```python
from build123d import *

# Parameters (mm, degrees)
SKETCH1_R           = 4.826
SKETCH1_R_2         = 4.064
SKETCH3_R           = 4.826
BOSS_EXTRUDE1_DEPTH = 2.54
BOSS_EXTRUDE1_DRAFT = -37
SKETCH5_R           = 4.826
BOSS_EXTRUDE2_DEPTH = 2.54
BOSS_EXTRUDE2_DRAFT = -37


with BuildPart() as part:
    # Sweep1: sweep along a path in Sketch2
    with BuildLine(Plane.XY) as sweep1_path:
        Line((0, 0), (0, 12.7))
        ThreePointArc((0, 12.7), (1.450094906, 19.990119387), (5.579615818, 26.170384182))
        Line((5.579615818, 26.170384182), (10.295384182, 30.886152545))
        ThreePointArc((10.295384182, 30.886152545), (15.875, 44.356536726), (10.295384182, 57.826920908))
        Line((10.295384182, 57.826920908), (5.579615818, 62.542689271))
        ThreePointArc((5.579615818, 62.542689271), (1.450094906, 68.722954066), (0, 76.013073453))
        Line((0, 76.013073453), (0, 88.713073453))
    # Sketch1 → Sweep1 (sweep)
    with BuildSketch(Plane(origin=(0, 0, 0), x_dir=(1, 0, 0), z_dir=(0, 1, 0))):
        Circle(SKETCH1_R)
        Circle(SKETCH1_R_2, mode=Mode.SUBTRACT)
    sweep(path=sweep1_path.line)


with BuildPart() as boss_extrude1_tool:
    # Sketch3 → Boss-Extrude1 (with draft: the straight prism first)
    with BuildSketch(Plane.XZ):
        with Locations(Location((0, 0, 0), (0, 0, 180))):
            Circle(SKETCH3_R)
    extrude(amount=BOSS_EXTRUDE1_DEPTH)
    # Boss-Extrude1: the draft: its side faces are tilted about the plane it starts from
    boss_extrude1_sides = [boss_extrude1_tool.faces().sort_by_distance(p)[0] for p in [
        (4.826, -1.27, 0),
    ]]
    draft(boss_extrude1_sides, Plane.XZ, BOSS_EXTRUDE1_DRAFT)


with BuildPart() as part_1:
    add(part.part)

    # Boss-Extrude1: add boss_extrude1_tool
    add(boss_extrude1_tool.part)

    # Cut-Extrude1 cone 1 section (through the dimple's axis) → Cut-Extrude1 (revolve, cut)
    with BuildSketch(Plane(origin=(0, -2.54, 0), x_dir=(0, 0, -1), z_dir=(1, 0, 0))):
        Polygon((0, 0), (5.978027287, 0), (0, 7.933110155), align=None)
    revolve(axis=Axis((0, -2.54, 0), (0, 1, 0)), mode=Mode.SUBTRACT)


with BuildPart() as boss_extrude2_tool:
    # Sketch5 → Boss-Extrude2 (with draft: the straight prism first)
    with BuildSketch(Plane(origin=(0, 88.713073453, 0), x_dir=(0, 0, -1), z_dir=(0, 1, 0))):
        with Locations(Location((0, 0, 0), (0, 0, 90))):
            Circle(SKETCH5_R)
    extrude(amount=BOSS_EXTRUDE2_DEPTH)
    # Boss-Extrude2: the draft: its side faces are tilted about the plane it starts from
    boss_extrude2_sides = [boss_extrude2_tool.faces().sort_by_distance(p)[0] for p in [
        (4.826, 89.983073453, 0),
    ]]
    draft(boss_extrude2_sides, Plane(origin=(0, 88.713073453, 0), x_dir=(0, 0, -1), z_dir=(0, 1, 0)), BOSS_EXTRUDE2_DRAFT)


with BuildPart() as part_2:
    add(part_1.part)

    # Boss-Extrude2: add boss_extrude2_tool
    add(boss_extrude2_tool.part)

    # Cut-Extrude2 cone 1 section (through the dimple's axis) → Cut-Extrude2 (revolve, cut)
    with BuildSketch(Plane(origin=(0, 91.253073453, 0), x_dir=(0, 0, 1), z_dir=(1, 0, 0))):
        Polygon((0, 0), (5.978027287, 0), (0, 7.933110155), align=None)
    revolve(axis=Axis((0, 91.253073453, 0), (0, -1, 0)), mode=Mode.SUBTRACT)


solid = part_2.part
```
Part model, mm, in its own coordinate system. A direction names the side the tool comes from. Round coordinates to 2 decimals unless told otherwise and drop trailing zeros. Write each loop counter-clockwise with the first axis right and the second up, starting at its lowest first coordinate (ties: lowest second). Pieces come first, ordered by that corner, then holes. Notation, with made-up numbers: (43, -21) -> (47, -21) arc R22 ccw to (47, 7) -> close; hole circle Ø4 at (49, -10). An arc over 180 degrees is marked (long way). Return JSON: item names as keys, results as strings. Group by question number.
Q1. Pin check, flat tips, straight feed: pin 1 (4 mm diameter, centred on y = 64, z = 3.5, fed in from +X); pin 2 (2 mm diameter, centred on y = 21, z = -5, fed in from -X); pin 3 (1 mm diameter, centred on x = 7.5, z = 3.5, fed in from +Y); pin 4 (8 mm diameter, centred on x = 0.5, z = -3.5, fed in from -Y). Stop position of each tip, or through.
Q2. Saw through at A-A on x = 10.25. State how many separate pieces and enclosed holes the cut face has, plus the area to 3 significant figures.
Q3. Which spindle directions (+Z, -Z, +X, -X, +Y, -Y) get a long thin tool onto all of the face, cutting with end or side? Do faces 5 (the cylindrical face through (-3.83, 6.439, 2.937)), 6 (the conical face through (1.592, 88.836, 3.84)), 7 (the cylindrical face through (-0.881, 6.439, 3.967)). Say none if no direction does.
Q4. Saw through at B-B on y = 85. Write the cut outline in (x, z).
Q5. Probe L1, parallel to X at y = 84.75, z = 0; L2, parallel to Y at x = 2.25, z = -3. List the from-to ranges inside material, lowest first. Write a range as [from, to].
Q6. Mould opens along Z. For faces 1 (the cylindrical face through (9.74, 62.05, -4.07)), 2 (the cylindrical face through (-0.881, 82.452, 3.967)), 3 (the cylindrical face through (10.7, 25.8, -1.2)), 4 (the flat face through (4, -2.54, 5)) say: pulls with the +Z half, pulls with the -Z half, needs draft (parallel to the pull), parting line crosses it, or undercut.
Answer:
{
 "1": {"pin 1": "x = 11.72", "pin 2": "x = -1.1", "pin 3": "y = 66.26", "pin 4": "y = -2.54"},
 "2": {"separate pieces": "2", "enclosed holes": "2", "area": "71.3 mm2"},
 "3": {"face 5": "none", "face 6": "+Y", "face 7": "-Y"},
 "4": {"outline": "circle Ø9.65 at (0, 0); hole circle Ø8.13 at (0, 0)"},
 "5": {"L1": "[-4.83, -4.06], [4.06, 4.83]", "L2": "[26.58, 28.16], [60.55, 62.13]"},
 "6": {"face 1": "parting line crosses it", "face 2": "undercut", "face 3": "undercut", "face 4": "needs draft"}
}
